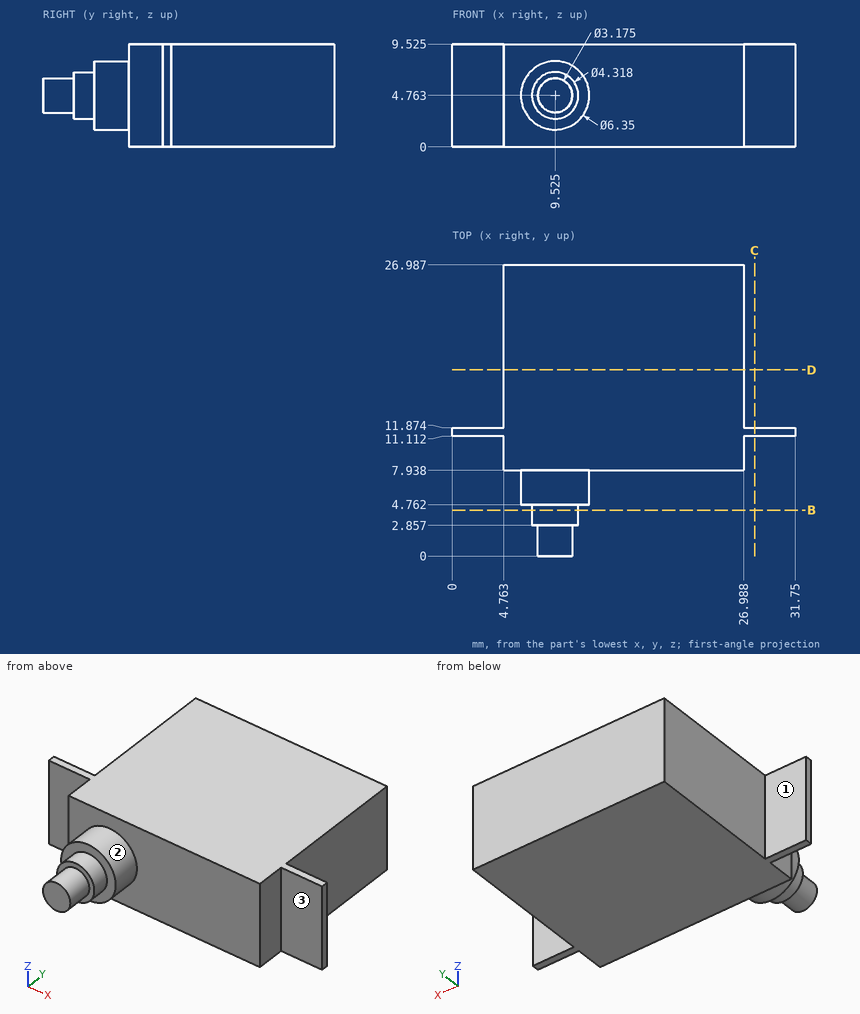
Here's the drawing with two shaded views (mm, measured from the low corner). I have some questions. A direction names the side the tool comes from. Coordinates: 2 decimals unless noted, no trailing zeros. Write each loop counter-clockwise with the first axis right and the second up, starting at its lowest first coordinate (ties: lowest second). Pieces come first, ordered by that corner, then holes.
Item 1: I want a section at C-C on x = 28. Write out the boundary of the cut face in (y, z) (1 decimal).
Item 2: Will these pins go through, and if not, where does the flat tip stop? pin 1 (2.5 mm diameter, centred on x = 2, z = 4, fed in from +Y) (1 decimal); pin 2 (1.5 mm diameter, centred on y = 3, z = 6.5, fed in from +X) (1 decimal); pin 3 (1 mm diameter, centred on y = 21, z = 5.5, fed in from +X).
Item 3: I want a section at D-D on y = 17.25. Write out the boundary of the cut face in (x, z) (1 decimal).
Item 4: I want a section at B-B on y = 4.25. Write out the boundary of the cut face in (x, z) (1 decimal).
Item 5: On a 3-axis mill with a long thin cutter (end or side, diameter ignored), from which of +Z, -Z, +X, -X, +Y, -Y can I reach the whole of each face in a straight line? I mean the marked faces 1, 2 and 3. Say none if no direction works.
Item 6: If I drill on line 1 (Y direction, x = 2.5, z = 3) (1 decimal); line 2 (X direction, y = 19, z = 6.5), over which ranges is the centre line in solid material (lowest first)?
Findings below:
1. outline: (11.1, 0) - (11.9, 0) - (11.9, 9.5) - (11.1, 9.5) - close
2. pin 1: stops at y = 11.9
2. pin 2: stops at x = 11.4
2. pin 3: stops at x = 26.99
3. outline: (4.8, 0) - (27, 0) - (27, 9.5) - (4.8, 9.5) - close
4. outline: circle Ø4.3 at (9.5, 4.8)
5. face 1: +Z, -Z, -X, +Y
5. face 2: -Y
5. face 3: +Z, -Z, +X, -Y
6. line 1: y = 11.1 to 11.9
6. line 2: x = 4.76 to 26.99
